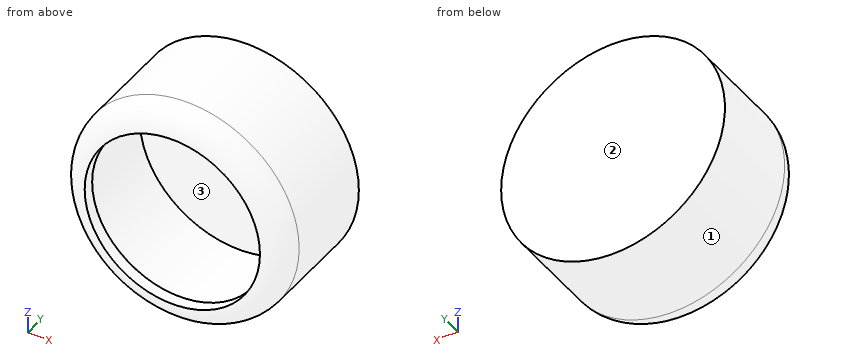
```python
from build123d import *

# Parameters (mm, degrees)
F2_R     = 23.428989388
F3_DEPTH = 25.4
F4_R     = 5.08
F5_T     = -2.54


# Not quite as in the source:
# - a shell that OpenCascade refuses in one call is made with other operations: the cavity is built on its own and cut out
# - the program builds the solid bodies; features that only make, move or delete a surface that nothing else refers to are left out


with BuildPart() as f3:
    # F2 (on Front) → F3 (new body)
    with BuildSketch(Plane.XZ):
        with Locations((0, 28.4662228078)):
            Circle(F2_R)
    extrude(amount=F3_DEPTH)

    # F4
    f4_edges = [f3.edges().sort_by_distance(p)[0] for p in [
        (-23.428989, -25.4, 28.466223),
    ]]
    fillet(f4_edges, radius=F4_R)

    # F5: a shell. OpenCascade refuses it in one call, so the cavity is built on its own and cut out:
    # the body offset inwards by the wall thickness, plus a prism from it out through each open face.
    f5_core = offset(f3.part, amount=F5_T, mode=Mode.PRIVATE)
    f5_exits = [f5_core.faces().sort_by_distance(p)[0] for p in [
        (0, -22.86, 28.466223),
    ]]
    add(f5_core, mode=Mode.SUBTRACT)
    extrude(f5_exits, amount=-F5_T, mode=Mode.SUBTRACT)


solid = f3.part
```
CAD build for the part. Positions are in the model's coordinates, mm. Face numbers are marked on the shaded views. Round coordinates to 2 decimals unless told otherwise and drop trailing zeros. Order: outer loops, then holes, each group sorted by start corner. A loop starts at its lowest first (then second) coordinate and runs counter-clockwise, first axis right, second up.
Q1. Two-plate mould, pull along Z, no slides. Class the marked faces 1, 2 and 3: pulls with the +Z half, pulls with the -Z half, needs draft (parallel to the pull), parting line crosses it, or undercut.
Q2. Drop flat-ended pins along their axis: pin 1 (4 mm diameter, centred on x = 2, y = -19.5, fed in from +Z); pin 2 (10 mm diameter, centred on y = -19, z = 39, fed in from +X); pin 3 (12 mm diameter, centred on x = -1, z = 24.5, fed in from -Y). Give the stop position or say it passes through.
Q3. Wall check: L1, parallel to Z at x = 0, y = -11.5; L2, parallel to Y at x = 14.5, z = 21; L3, parallel to Z at x = -15.5, y = -2.75. Give the ranges that are in metal, low to high.
Q4. Slice it at A-A (x = 0). Write the cut outline in (y, z).
Q5. Slice it at B-B (y = -12.25). Write the cut outline in (x, z).
Results below:
1. face 1: parting line crosses it
1. face 2: needs draft
1. face 3: undercut
2. pin 1: stops at z = 51.9
2. pin 2: stops at x = 22.77
2. pin 3: stops at y = -2.54
3. L1: z = 5.04 to 7.58, 49.36 to 51.9
3. L2: y = -2.54 to 0
3. L3: z = 10.9 to 14.46, 42.47 to 46.04
4. outline: (-25.4, 10.12) arc R5.08 ccw to (-20.32, 5.04) - (0, 5.04) - (0, 51.9) - (-20.32, 51.9) arc R5.08 ccw to (-25.4, 46.82) - (-22.86, 46.82) arc R2.54 cw to (-20.32, 49.36) - (-2.54, 49.36) - (-2.54, 7.58) - (-20.32, 7.58) arc R2.54 cw to (-22.86, 10.12) - close
5. outline: circle Ø46.86 at (0, 28.47); hole circle Ø41.78 at (0, 28.47)
